Verification items for the finished model (mm, model axes). Face numbers are marked on the shaded views. A direction names the side the tool comes from. Give positions to 0.01 mm unless a question says otherwise; leave off trailing zeros. Order: outer loops, then holes, each group sorted by start corner. A loop starts at its lowest first (then second) coordinate and runs counter-clockwise, first axis right, second up. Notation, with made-up numbers: (-34.75, 15) -> (-12.75, 15) arc R24 cw to (-12.75, 43) -> close; hole circle Ø4 at (46, -10). An arc over 180 degrees is marked (long way). Return JSON: item names as keys, results as strings. Group by question number.
(1) Tool access check on the marked faces 5 and 6. Record the directions out of +Z, -Z, +X, -X, +Y, -Y that give a thin tool (end or side, any length) a straight path to the whole face; none if there is none.
(2) Cross-section at C-C on z = 3. Enter the section's corners in (x, y).
(3) Release check for a two-part mould opening along X. For the marked faces 1, 2, 3 and 4 record: pulls with the +X half, pulls with the -X half, needs draft (parallel to the pull), parting line crosses it, or undercut.
(4) Cross-section at D-D on y = -4.5. Enter the section's corners in (x, z).
(5) Depth check by flat-ended pin: pin 1 Ø1.5 at (x, y) = (-6, -3.5) entering from +Z; pin 2 Ø5.5 at (x, z) = (-6.5, 16) entering from -Y; pin 3 Ø3 at (x, y) = (-3, 1.5) entering from +Z. Enter the tip coordinate at first touch or a pass-through.
(6) Thickness scan on line 1 along Y through (x, z) = (-11.25, 18.25); line 2 along Y through (x, z) = (3, 9); line 3 along Z through (x, y) = (-1.75, 2.5). Record the ranges inside material, lowest first.
(7) Cross-section at B-B on y = 7.25. Enter the section's corners in (x, z), then the cut area to 3 significant figures.
(8) Cross-section at A-A on x = 8. Enter the section's corners in (y, z), then the cut area to 3 significant figures.
from build123d import *

# Parameters (mm, degrees)
EXTRUDE_3_DEPTH = 13
SKETCH_5_4_W    = 28
SKETCH_5_4_H    = 10.634799235
EXTRUDE_4_DEPTH = 13
EXTRUDE_5_DEPTH = 7


with BuildPart() as part:
    # Sketch 5 → Extrude 3 (new body)
    with BuildSketch(Plane.XY):
        with BuildLine():
            Line((14, 9), (5, 9))
            ThreePointArc((5, 9), (0, 4), (-5, 9))
            Line((-5, 9), (-14, 9))
            Line((-14, 9), (-14, 1.634799235))
            Line((-14, 1.634799235), (14, 1.634799235))
            Line((14, 1.634799235), (14, 9))
        make_face()
    extrude(amount=EXTRUDE_3_DEPTH)



with BuildPart() as body_2:
    # Sketch 5_4 → Extrude 4 (new body)
    with BuildSketch(Plane.XY):
        with Locations((0, -3.682600382)):
            Rectangle(SKETCH_5_4_W, SKETCH_5_4_H)
    extrude(amount=EXTRUDE_4_DEPTH)


with BuildPart() as part_1:
    add(part.part)

    add(body_2.part)  # Extrude 5 merges body 2
    # Sketch 6 → Extrude 5 (add)
    with BuildSketch(Plane.XY.offset(13)):
        with BuildLine():
            Line((14, 9), (10, 9))
            ThreePointArc((10, 9), (9.155369145, 4.977660404), (6.764156835, 1.634799235))
            Line((6.764156835, 1.634799235), (14, 1.634799235))
            Line((14, 1.634799235), (14, 9))
        make_face()
        with BuildLine():
            Line((-6.764156835, 1.634799235), (-14, 1.634799235))
            Line((-14, 1.634799235), (-14, -3))
            Line((-14, -3), (14, -3))
            Line((14, -3), (14, 1.634799235))
            Line((14, 1.634799235), (6.764156835, 1.634799235))
            ThreePointArc((6.764156835, 1.634799235), (0, -1), (-6.764156835, 1.634799235))
        make_face()
        with BuildLine():
            Line((-10, 9), (-14, 9))
            Line((-14, 9), (-14, 1.634799235))
            Line((-14, 1.634799235), (-6.764156835, 1.634799235))
            ThreePointArc((-6.764156835, 1.634799235), (-9.155369145, 4.977660404), (-10, 9))
        make_face()
    extrude(amount=EXTRUDE_5_DEPTH)


solid = part_1.part
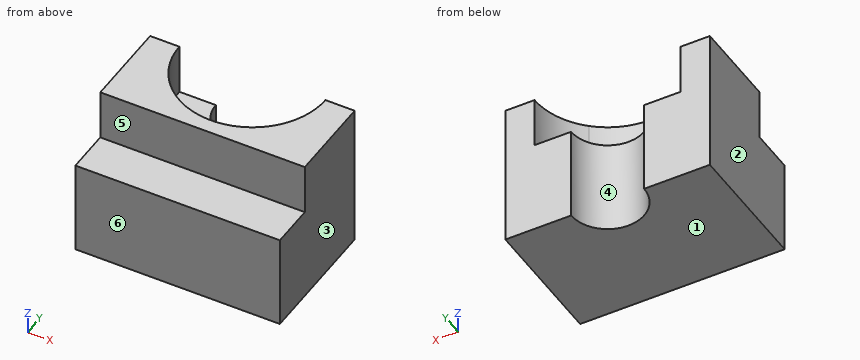
Verdict:
{
 "1": {"face 5": "+Z, +X, -X, -Y", "face 6": "+Z, -Z, +X, -X, -Y"},
 "2": {"outline": "(-14, -9) -> (14, -9) -> (14, 9) -> (5, 9) arc R5 cw to (-5, 9) -> (-14, 9) -> close"},
 "3": {"face 1": "needs draft", "face 2": "pulls with the -X half", "face 3": "pulls with the +X half", "face 4": "undercut"},
 "4": {"outline": "(-14, 0) -> (14, 0) -> (14, 13) -> (-14, 13) -> close"},
 "5": {"pin 1": "z = 20", "pin 2": "y = -3", "pin 3": "z = 13"},
 "6": {"line 1": "-3 to 9", "line 2": "-9 to 5", "line 3": "0 to 13"},
 "7": {"outline": "(-14, 0) -> (-4.68, 0) -> (-4.68, 13) -> (-9.85, 13) -> (-9.85, 20) -> (-14, 20) -> close; (4.68, 0) -> (14, 0) -> (14, 20) -> (9.85, 20) -> (9.85, 13) -> (4.68, 13) -> close", "area": "300 mm²"},
 "8": {"outline": "(-9, 0) -> (9, 0) -> (9, 13) -> (3, 13) -> (3, 20) -> (-3, 20) -> (-3, 13) -> (-9, 13) -> close", "area": "276 mm²"}
}
